The model under review builds one solid part; all positions refer to its coordinate system, in mm. A direction names the side the tool comes from. Coordinates: 2 decimals unless noted, no trailing zeros. Order: outer loops, then holes, each group sorted by start corner. A loop starts at its lowest first (then second) coordinate and runs counter-clockwise, first axis right, second up. Notation, with made-up numbers: (-31.75, -1.5) - (-12.75, -1.5) arc R30 ccw to (-12.75, 35.5) - close; hole circle Ø4 at (3, 42). An arc over 180 degrees is marked (long way). Answer in a Markdown table with one row per item.
```python
from build123d import *

# Parameters (mm, degrees)
ESQUISSE1_R        = 6
BOSS_EXTRU_1_DEPTH = 3
ESQUISSE2_R        = 8
ESQUISSE2_R_2      = 6
BOSS_EXTRU_2_DEPTH = 2


with BuildPart() as part:
    # Esquisse1 → Boss.-Extru.1 (new, symmetric)
    with BuildSketch(Plane.XY):
        Circle(ESQUISSE1_R)
        with BuildLine():
            ThreePointArc((-0.642168668, 1.999404762), (-1.48492424, -1.48492424), (1.999404762, -0.642168668))
            ThreePointArc((1.999404762, -0.642168668), (2.75, 0), (1.999404762, 0.642168668))
            ThreePointArc((1.999404762, 0.642168668), (1.48492424, 1.48492424), (0.642168668, 1.999404762))
            ThreePointArc((0.642168668, 1.999404762), (0, 2.75), (-0.642168668, 1.999404762))
        make_face(mode=Mode.SUBTRACT)
    extrude(amount=BOSS_EXTRU_1_DEPTH, both=True)

    # Esquisse2 → Boss.-Extru.2 (add)
    with BuildSketch(Plane.XY.offset(3)):
        Circle(ESQUISSE2_R)
        Circle(ESQUISSE2_R_2, mode=Mode.SUBTRACT)
    boss_extru_2 = extrude(amount=-BOSS_EXTRU_2_DEPTH)

    # Symétrie1: Boss.-Extru.2 across plane
    add(boss_extru_2.mirror(Plane.XY))


solid = part.part
```
Item 1: Clearance check with flat-ended pins moving along their axes: pin 1 Ø1.5 at (y, z) = (1.5, -1.5) entering from +X; pin 2 Ø2 at (x, z) = (2, -1) entering from +Y; pin 3 Ø2 at (y, z) = (-4.5, -1) entering from -X. State where each tip first meets the part, or that it passes through.
Check values:
| item | result |
|---|---|
| pin 1 | x = 7.96 |
| pin 2 | y = 7.94 |
| pin 3 | x = -7.19 |
Item 2: To check wall thickness, follow line 1 (Z direction, x = 6.5, y = -4.5); line 2 (Y direction, x = 0, z = 0.15); line 3 (Y direction, x = 2.1, z = -0.65). State the ranges of each line that lie inside material, in increasing order. Write a range as from..to.
Check values:
| item | result |
|---|---|
| line 1 | -3..-1, 1..3 |
| line 2 | -6..-2.1, 2.75..6 |
| line 3 | -5.62..-0.65, 0.65..5.62 |
Item 3: We need section A-A, the plane y = 0. Write out the cut boundary in (x, z), then the cut area to 3 significant figures.
Check values:
| item | result |
|---|---|
| outline | (-8, -3) - (-2.1, -3) - (-2.1, 3) - (-8, 3) - (-8, 1) - (-6, 1) - (-6, -1) - (-8, -1) - close; (2.75, -3) - (8, -3) - (8, -1) - (6, -1) - (6, 1) - (8, 1) - (8, 3) - (2.75, 3) - close |
| area | 58.9 mm^2 |
Item 4: Mouldability with a two-part tool opening along X and no side actions: class faces 1 (the face through (-1.73, -7.81, -2.01)), 2 (the face through (-2, 6, -1)), 3 (the face through (1.49, 1.48, 0.04)) as +X half, -X half, draft (parallel to the pull), parting line (faces both ways), or undercut.
Check values:
| item | result |
|---|---|
| face 1 | parting line |
| face 2 | draft |
| face 3 | undercut |
Item 5: Tool access review of faces 4 (the face through (2, -2, 3)), 5 (the face through (-2, 6, 1)): name each direction out of +Z, -Z, +X, -X, +Y, -Y from which nothing blocks a thin tool from reaching the whole face with its end or side.
Check values:
| item | result |
|---|---|
| face 4 | +Z, +X, -X, +Y, -Y |
| face 5 | none |
Item 6: We need section C-C, the plane z = -0.5. Write out the cut boundary in (x, y), then the cut area to 3 significant figures.
Check values:
| item | result |
|---|---|
| outline | circle Ø12 at (0, 0); hole (-0.64, 2) arc R2.1 ccw (long way) to (2, -0.64) arc R0.65 ccw (long way) to (2, 0.64) arc R2.1 ccw to (0.64, 2) arc R0.65 ccw (long way) to start |
| area | 97.8 mm^2 |
Item 7: We need section D-D, the plane x = 5.5. Write out the cut boundary in (y, z), then the cut area to 3 significant figures.
Check values:
| item | result |
|---|---|
| outline | (-5.81, -3) - (5.81, -3) - (5.81, -1) - (2.4, -1) - (2.4, 1) - (5.81, 1) - (5.81, 3) - (-5.81, 3) - (-5.81, 1) - (-2.4, 1) - (-2.4, -1) - (-5.81, -1) - close |
| area | 56.1 mm^2 |
